Geometry: final body of the model. Coordinates: model frame, mm. A direction names the side the tool comes from. Give positions to 0.01 mm unless a question says otherwise; leave off trailing zeros. Loops run counter-clockwise (first coordinate to the right, second up) from the corner with the lowest first, then second, coordinate; pieces in that order, holes last.
Autodesk Inventor part; units mm, degrees
ref_plane "YZ Plane" through (0, 0, 0) normal (1, 0, 0) x (0, 1, 0)
ref_plane "XZ Plane" through (0, 0, 0) normal (0, 1, 0) x (-1, 0, 0)
ref_plane "XY Plane" through (0, 0, 0) normal (0, 0, 1) x (1, 0, 0)
sketch "Szkic1" plane through (0, 0, 0) normal (0, 0, 1) x (1, 0, 0)
  line L0 (-2.5, 0) -> (-27.5, 0)
  line L1 (-27.5, 0) -> (-19.7354, -28.9778)
  line L2 (-27.5, 0) -> (2.5, 0) construction
  line L3 (-27.5, 0) -> (-37.3351, 36.7052)
  line L4 (-27.5, 0) -> (10.5, 0) construction
  line L5 (-37.3351, 36.7052) -> (-37.3351, 54.7052)
  line L6 (-37.3351, 54.7052) -> (-2.5, 54.7052)
  line L7 (-37.3351, 54.7052) -> (-27.3351, 72.0257)
  line L8 (-37.3351, 54.7052) -> (-17.3351, 54.7052) construction
  line L9 (-37.3351, 54.7052) -> (-27.3351, 37.3847)
  line L10 (-37.3351, 54.7052) -> (-17.3351, 54.7052) construction
  circle A0 centre (-27.5, 0) radius 1.5
  line L11 (-2.5, 0) -> (-2.5, -12)
  line L12 (-2.5, -12) -> (-27.5, -12)
  line L13 (-27.5, -12) -> (-19.7354, -28.9778)
  line L14 (-27.5, -12) -> (-48.0171, 32.862)
  line L15 (-48.0171, 32.862) -> (-51.0127, 50.611)
  line L16 (-48.0171, 32.862) -> (-30.0171, 32.862) construction
  line L17 (-51.0127, 50.611) -> (-38.2696, 35.1962)
  line L18 (-51.0127, 50.611) -> (-31.0127, 50.611) construction
  line L19 (-51.0127, 50.611) -> (-44.0347, 69.3542)
  line L20 (-51.0127, 50.611) -> (-31.0127, 50.611) construction
  circle A1 centre (-27.5, -12) radius 1.5
  line L21 (-19.7354, -28.9778) -> (0, -28.9778)
  circle A2 centre (-19.7354, -28.9778) radius 2.5
  line L22 (-22.2354, -28.9778) -> (-27.2354, -28.9778)
  line L23 (17.2354, -28.9778) -> (22.2354, -28.9778)
  circle A3 centre (14.7354, -28.9778) radius 2.5
  line L24 (22.5, -12) -> (14.7354, -28.9778)
  line L25 (14.7354, -28.9778) -> (0, -28.9778)
  line L26 (-2.5, -12) -> (22.5, -12)
  line L27 (32.3351, 54.7052) -> (22.3351, 37.3847)
  line L28 (32.3351, 36.7052) -> (32.3351, 54.7052)
  line L29 (46.0127, 50.611) -> (33.2696, 35.1962)
  line L30 (43.0171, 32.862) -> (46.0127, 50.611)
  line L31 (43.0171, 32.862) -> (25.0171, 32.862) construction
  circle A4 centre (22.5, 0) radius 1.5
  line L32 (22.5, 0) -> (32.3351, 36.7052)
  circle A5 centre (22.5, -12) radius 1.5
  line L33 (22.5, -12) -> (43.0171, 32.862)
  line L34 (-2.5, 0) -> (22.5, 0)
  line L35 (22.5, 0) -> (14.7354, -28.9778)
  line L36 (22.5, 0) -> (-7.5, 0) construction
  line L37 (22.5, 0) -> (-15.5, 0) construction
  line L38 (46.0127, 50.611) -> (26.0127, 50.611) construction
  line L39 (46.0127, 50.611) -> (26.0127, 50.611) construction
  line L40 (32.3351, 54.7052) -> (12.3351, 54.7052) construction
  line L41 (32.3351, 54.7052) -> (12.3351, 54.7052) construction
  line L42 (32.3351, 54.7052) -> (-2.5, 54.7052)
  line L43 (46.0127, 50.611) -> (39.0347, 69.3542)
  line L44 (32.3351, 54.7052) -> (22.3351, 72.0257)
  line L45 (-19.7354, -31.4778) -> (-19.7354, -36.4778)
  line L46 (-19.7354, -36.4778) -> (0, -36.4778)
  line L47 (-19.7354, -36.4778) -> (-22.2354, -36.4778)
  line L48 (-27.2354, -28.9778) -> (-27.2354, -31.4778)
  line L49 (-19.7354, -26.4778) -> (-19.7354, -21.4778)
  line L50 (-19.7354, -21.4778) -> (-22.2354, -21.4778)
  line L51 (-27.2354, -26.4778) -> (-27.2354, -28.9778)
  line L52 (-19.7354, -21.4778) -> (0, -21.4778)
  line L53 (22.5, 0) -> (14.7354, -28.9778)
  line L54 (22.5, -12) -> (14.7354, -28.9778)
  line L55 (14.7354, -28.9778) -> (-5, -28.9778)
  circle A6 centre (14.7354, -28.9778) radius 2.5
  line L56 (17.2354, -28.9778) -> (22.2354, -28.9778)
  line L57 (-19.7354, -28.9778) -> (-5, -28.9778)
  line L58 (14.7354, -31.4778) -> (14.7354, -36.4778)
  line L59 (14.7354, -36.4778) -> (-5, -36.4778)
  line L60 (14.7354, -36.4778) -> (17.2354, -36.4778)
  line L61 (22.2354, -28.9778) -> (22.2354, -31.4778)
  line L62 (14.7354, -26.4778) -> (14.7354, -21.4778)
  line L63 (14.7354, -21.4778) -> (17.2354, -21.4778)
  line L64 (22.2354, -26.4778) -> (22.2354, -28.9778)
  line L65 (14.7354, -21.4778) -> (-5, -21.4778)
  arc A7 (-22.2354, -21.4778) -> (-27.2354, -26.4778) centre (-22.2354, -26.4778) ccw
  arc A8 (-27.2354, -31.4778) -> (-22.2354, -36.4778) centre (-22.2354, -31.4778) ccw
  arc A9 (22.2354, -26.4778) -> (17.2354, -21.4778) centre (17.2354, -26.4778) ccw
  arc A10 (17.2354, -36.4778) -> (22.2354, -31.4778) centre (17.2354, -31.4778) ccw
  point P0 (0, 0)
  point P1 (-27.2354, -36.4778)
  point P2 (-27.2354, -21.4778)
  point P3 (22.2354, -36.4778)
  point P4 (22.2354, -21.4778)
  dimension "d0" = 25
  dimension "d1" = 30
  dimension "d2" = 75
  dimension "d3" = 38
  dimension "d4" = 105
  dimension "d5" = 18
  dimension "d6" = 20
  dimension "d7" = 60
  dimension "d8" = 20
  dimension "d9" = 60
  dimension "d10" = 3
  dimension "d11" = 12
  dimension "d12" = 25
  dimension "d13" = 49.331
  dimension "d14" = 18
  dimension "d15" = 99.58
  dimension "d16" = 20
  dimension "d17" = 50.42
  dimension "d18" = 20
  dimension "d19" = 69.58
  dimension "d20" = 3
  dimension "d22" = 5
  dimension "d23" = 5
  dimension "d28" = 5
  dimension "d29" = 5
  dimension "d30" = 5
  dimension "d31" = 5
  dimension "d32" = 5
  dimension "d33" = 5
extrude "Wyciągnięcie proste1" add sketch "Szkic1" along normal mid plane 10 contours L50 L49 A2 L1 | L1 A2 L13 A7 L50 | L63 A9 L24 A3 L35 | L35 A3 L62 L63 | L52 L65 L62 A3 L25 L21 A2 L49 | A2 L22 L51 A7 L13 | A9 L64 L23 A3 L24 | L21 L25 A3 L58 L59 L46 L45 A2 | A2 L45 L47 A8 L48 L22 | L23 L61 A10 L60 L58 A3
sketch "Szkic2" plane through (0, 0, 5) normal (0, 0, 1) x (1, 0, 0)
  circle A0 centre (-19.7354, -28.9778) radius 2.5
  circle A1 centre (-19.7354, -28.9778) radius 2.5
  circle A2 centre (14.7354, -28.9778) radius 2.5
  circle A3 centre (14.7354, -28.9778) radius 2.5
  point P0 (0, 0)
extrude "Wyciągnięcie proste2" add sketch "Szkic2" along normal blind 10 and the other way blind 20
sketch "Szkic3" plane through (-22.2354, -36.4778, 5) normal (0, -1, 0) x (1, 0, 0)
  line L0 (44.4709, -10) -> (44.4709, 0)
  line L1 (44.4709, -5) -> (-5, -5)
  line L2 (-5, -10) -> (-5, 0)
  line L3 (0, 0) -> (39.4709, 0)
  line L4 (19.7354, 0) -> (19.7354, -10)
  circle A0 centre (19.7354, -5) radius 1.6
  point P0 (22.2354, -5)
  dimension "d40" = 3.2
extrude "Wyciągnięcie proste3" cut sketch "Szkic3" against normal through all
sketch "Szkic4" plane through (14.7354, -28.9778, 15) normal (0, 0, 1) x (1, 0, 0)
  circle A0 centre (0, 0) radius 2.5
  circle A1 centre (-34.4709, 0) radius 2.5
  circle A2 centre (-34.4709, 0) radius 2.5
  point P0 (-14.7354, 28.9778)
extrude "Wyciągnięcie proste4" cut sketch "Szkic4" against normal through all
sketch "Szkic5" plane through (0, 0, 5) normal (0, 0, 1) x (1, 0, 0)
  line L0 (-22.2354, -21.4778) -> (17.2354, -21.4778)
  line L1 (0, -21.4778) -> (0, -22.7258)
  line L2 (0, -21.4778) -> (1.248, -21.4778) construction
  circle A0 centre (14.7354, -28.9778) radius 2.5
  circle A1 centre (14.7354, -28.9778) radius 7.5
  circle A2 centre (-19.7354, -28.9778) radius 2.5
  circle A3 centre (-19.7354, -28.9778) radius 7.5
  line L3 (0, -22.7258) -> (7.2354, -22.7258)
  line L4 (7.2354, -22.7258) -> (7.2354, -28.9778)
  line L5 (0, -22.7258) -> (-12.2354, -22.7258)
  line L6 (-12.2354, -22.7258) -> (-12.2354, -28.9778)
  line L7 (22.2354, -28.9778) -> (22.2354, -21.4778)
  line L8 (22.2354, -26.4778) -> (22.2354, -31.4778)
  line L9 (7.2354, -22.7258) -> (7.2354, -12.7258)
  line L10 (7.2354, -12.7258) -> (-12.2354, -12.7258)
  line L11 (-12.2354, -12.7258) -> (-27.2354, -12.7258)
  line L12 (-27.2354, -12.7258) -> (-27.2354, -28.9778)
  line L13 (22.2354, -21.4778) -> (22.2354, -12.7258)
  line L14 (22.2354, -12.7258) -> (7.2354, -12.7258)
  line L15 (-27.2354, -12.7258) -> (-27.2354, -17.7258)
  line L16 (-27.2354, -12.7258) -> (-27.2354, -17.7258)
  line L17 (-27.2354, -17.7258) -> (22.2354, -17.7258)
  point P0 (0, 0)
  dimension "d45" = 1.248
  dimension "d46" = 270
  dimension "d47" = 7.5
  dimension "d48" = 10
extrude "Wyciągnięcie proste5" add sketch "Szkic5" along normal blind 10 contours A3 L12 L17 L9 L0 | L0 L1 L5 L6 A3 | A3 | L0 L9 L3 L1 | L9 L17 L13 L7 A1 L0 | L0 A1 L4 L9 | A1
sketch "Szkic6" plane through (0, 0, -5) normal (0, 0, -1) x (-1, 0, 0)
  line L0 (22.2354, -21.4778) -> (-17.2354, -21.4778)
  arc A0 (-17.2354, -21.4778) -> (-22.2354, -26.4778) centre (-17.2354, -26.4778) ccw
  line L1 (-22.2354, -26.4778) -> (-22.2354, -31.4778)
  arc A1 (-22.2354, -31.4778) -> (-17.2354, -36.4778) centre (-17.2354, -31.4778) ccw
  line L2 (-17.2354, -36.4778) -> (22.2354, -36.4778)
  arc A2 (22.2354, -36.4778) -> (27.2354, -31.4778) centre (22.2354, -31.4778) ccw
  line L3 (27.2354, -31.4778) -> (27.2354, -26.4778)
  arc A3 (27.2354, -26.4778) -> (22.2354, -21.4778) centre (22.2354, -26.4778) ccw
  point P0 (0, 0)
extrude "Wyciągnięcie proste6" cut sketch "Szkic6" against normal blind 10
fillet "Zaokrąglenie1" radius 2 4 edges at (-12.2354, -22.7258, 10) (7.2354, -22.7258, 10) (22.2354, -17.7258, 10) (-27.2354, -17.7258, 10)
sketch "Szkic7" plane through (-25.2354, -17.7258, 5) normal (0, 1, 0) x (1, 0, 0)
  line L0 (15, -10) -> (30.4709, -10)
  line L1 (22.7354, -10) -> (28.8669, -10)
  line L2 (28.8669, -10) -> (28.8669, -16)
  line L3 (28.8669, -16) -> (16.6039, -16)
  line L4 (16.6039, -16) -> (16.6039, -10)
  line L5 (22.7354, -10) -> (16.6039, -10)
  line L6 (16.6039, -10) -> (16.6039, 0)
  line L7 (22.7354, 6) -> (28.8669, 6)
  line L8 (28.8669, 6) -> (28.8669, 0)
  line L9 (28.8669, 0) -> (16.6039, 0)
  line L10 (16.6039, 0) -> (16.6039, 6)
  line L11 (22.7354, 6) -> (16.6039, 6)
  point P0 (25.2354, 5)
  dimension "d54" = 6.1315
  dimension "d55" = 6
  dimension "d56" = 12.263
  dimension "d57" = 10
  dimension "d58" = 6.1315
  dimension "d59" = 6
  dimension "d60" = 12.263
extrude "Wyciągnięcie proste7" add sketch "Szkic7" against normal up to surface (5 mm away)
sketch "Szkic8" plane through (-25.2354, -17.7258, 15) normal (0, 1, 0) x (1, 0, 0)
  line L0 (28.8669, 16) -> (16.6039, 16)
  line L1 (22.7354, 16) -> (22.7354, -6)
  line L2 (16.6039, -6) -> (28.8669, -6)
  circle A0 centre (22.7354, 5) radius 1.6
  point P0 (25.2354, 15)
  dimension "d64" = 3.2
extrude "Wyciągnięcie proste8" cut sketch "Szkic8" against normal blind 10
sketch "Szkic9" plane through (-25.2354, -17.7258, 15) normal (0, 1, 0) x (1, 0, 0)
  point P0 (22.7354, 13.5)
hole "Otwór1" at (-2.5, -17.7258, 1.5) direction (0, -1, 0) diameter 2.9 end through all
sketch "Szkic10" plane through (-25.2354, -17.7258, 15) normal (0, 1, 0) x (1, 0, 0)
  point P0 (22.7354, -3.5)
hole "Otwór2" at (-2.5, -17.7258, 18.5) direction (0, -1, 0) diameter 2.9 end through all
sketch "Szkic11" plane through (-25.2354, -17.7258, 15) normal (0, 1, 0) x (1, 0, 0)
  circle A0 centre (22.7354, 5) radius 1.6
  circle A1 centre (22.7354, 5) radius 3.5
  point P0 (25.2354, 15)
  dimension "d81" = 7
extrude "Wyciągnięcie proste9" cut sketch "Szkic11" against normal blind 2
properties part number "Podstawa chwytaka" material "Stal, węglowa"
Item 1: Ray query, probe 1 along Z at (x, y) = (-2.5, -20); probe 2 along X at (y, z) = (-29, 7.25); probe 3 along Y at (x, z) = (-3, 17). Return the intervals inside material, ascending.
Values follow:
probe 1: z = -1 to 0.05, 2.95 to 8.4, 11.6 to 17.05, 19.95 to 21
probe 2: x = -27.24 to -22.24, -17.24 to -12.24, 7.24 to 12.24, 17.24 to 22.24
probe 3: y = -22.73 to -17.73
Item 2: Pin query (flat end, axial travel): pin 1 (5.5 mm diameter, centred on x = -20, y = -28, fed in from -Z); pin 2 (1.5 mm diameter, centred on y = -20.5, z = 3, fed in from +X); pin 3 (12 mm diameter, centred on x = -13.5, z = 12, fed in from -Y). Return the tip coordinate at first contact, or that it passes through.
Values follow:
pin 1: stops at z = 5
pin 2: stops at x = 3.63
pin 3: stops at y = -36.47
Item 3: Section query D-D on y = -19. Return loops of the section in (x, z), plus the area to 3 significant figures.
Values follow:
outline: (-27.1, 5) - (-8.63, 5) - (-8.63, -1) - (3.63, -1) - (3.63, 5) - (22.1, 5) - (22.1, 15) - (3.63, 15) - (3.63, 21) - (-8.63, 21) - (-8.63, 15) - (-27.1, 15) - close; hole circle Ø7 at (-2.5, 10); hole circle Ø2.9 at (-2.5, 1.5); hole circle Ø2.9 at (-2.5, 18.5)
area: 587 mm2
Item 4: Draft query along Z for faces 1 (the face through (-2, -20, 21)), 2 (the face through (6.67, -23.33, 10.07)), 3 (the face through (-2, -19.726, 12)). Return one class per face: +Z half, -Z half, draft (parallel to the pull), parting line (faces both ways), or undercut.
Values follow:
face 1: +Z half
face 2: draft
face 3: undercut
Item 5: Section query C-C on x = -2.5. Return loops of the section in (y, z).
Values follow:
outline: (-22.73, -1) - (-17.73, -1) - (-17.73, 0.05) - (-22.73, 0.05) - close; (-22.73, 2.95) - (-17.73, 2.95) - (-17.73, 6.5) - (-19.73, 6.5) - (-19.73, 8.4) - (-22.73, 8.4) - close; (-22.73, 11.6) - (-19.73, 11.6) - (-19.73, 13.5) - (-17.73, 13.5) - (-17.73, 17.05) - (-22.73, 17.05) - close; (-22.73, 19.95) - (-17.73, 19.95) - (-17.73, 21) - (-22.73, 21) - close
Item 6: Set-up query: faces 4 (the face through (15, -25, 15)), 5 (the face through (-8.632, -20, 2)), 6 (the face through (3.632, -20, 2)). Return all of +Z, -Z, +X, -X, +Y, -Y with unobstructed straight access to the full face (end or side cutting, diameter ignored); none if empty.
Values follow:
face 4: +Z, +X, +Y, -Y
face 5: -Z, -X, +Y, -Y
face 6: -Z, +X, +Y, -Y
Item 7: Section query A-A on z = 10. Return loops of the section in (x, y), plus the area to 3 significant figures.
Values follow:
outline: (-27.24, -28.98) arc R7.5 ccw to (-12.24, -28.98) - (-12.24, -24.73) arc R2 cw to (-10.24, -22.73) - (-4.1, -22.73) - (-4.1, -19.73) - (-6, -19.73) - (-6, -17.73) - (-25.24, -17.73) arc R2 ccw to (-27.24, -19.73) - close; (-0.9, -22.73) - (5.24, -22.73) arc R2 cw to (7.24, -24.73) - (7.24, -28.98) arc R7.5 ccw to (22.24, -28.98) - (22.24, -19.73) arc R2 ccw to (20.24, -17.73) - (1, -17.73) - (1, -19.73) - (-0.9, -19.73) - close; hole circle Ø5 at (-19.74, -28.98); hole circle Ø5 at (14.74, -28.98)
area: 549 mm2
Item 8: Section query B-B on z = 18.5. Return loops of the section in (x, y), plus the area to 3 significant figures.
Values follow:
outline: (-8.63, -22.73) - (-3.95, -22.73) - (-3.95, -17.73) - (-8.63, -17.73) - close; (-1.05, -22.73) - (3.63, -22.73) - (3.63, -17.73) - (-1.05, -17.73) - close
area: 46.8 mm2
